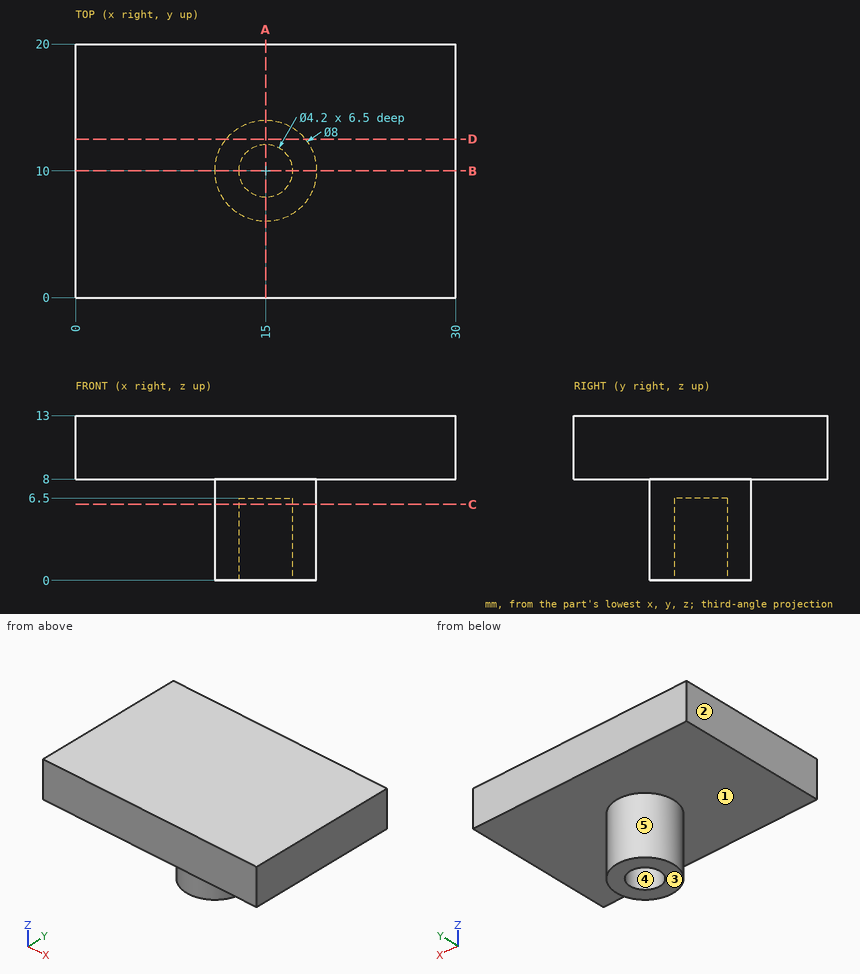
Source: three-view drawing plus pictorial views. Frame: mm from the lowest corner of the part. A direction names the side the tool comes from. Coordinates: 2 decimals unless noted, no trailing zeros. Order: outer loops, then holes, each group sorted by start corner. A loop starts at its lowest first (then second) coordinate and runs counter-clockwise, first axis right, second up.
1) Ray query, probe 1 along Y at (x, z) = (15, 4.5); probe 2 along Z at (x, y) = (22.5, 7.75); probe 3 along Z at (x, y) = (15, 10.5). Return the intervals inside material, ascending.
Result sheet:
probe 1: y = 6 to 7.9, 12.1 to 14
probe 2: z = 8 to 13
probe 3: z = 6.5 to 13
2) Section C-C (z = 6). Return loops of the section in (x, y).
Result sheet:
outline: circle Ø8 at (15, 10); hole circle Ø4.2 at (15, 10)
3) Section B-B (y = 10). Return loops of the section in (x, z), then the cut area to 3 significant figures.
Result sheet:
outline: (0, 8) - (11, 8) - (11, 0) - (12.9, 0) - (12.9, 6.5) - (17.1, 6.5) - (17.1, 0) - (19, 0) - (19, 8) - (30, 8) - (30, 13) - (0, 13) - close
area: 187 mm2
4) Draft query along Y for the marked faces 3, 4 and 5. Return one class per face: released by +Y, released by -Y, zero draft, split by the parting line, or undercut.
Result sheet:
face 3: zero draft
face 4: undercut
face 5: split by the parting line
5) Set-up query: the marked faces 1 and 2. Return all of +Z, -Z, +X, -X, +Y, -Y with unobstructed straight access to the full face (end or side cutting, diameter ignored); none if empty.
Result sheet:
face 1: -Z
face 2: +Z, -Z, -X, +Y, -Y
6) Section A-A (x = 15). Return loops of the section in (y, z), then the cut area to 3 significant figures.
Result sheet:
outline: (0, 8) - (6, 8) - (6, 0) - (7.9, 0) - (7.9, 6.5) - (12.1, 6.5) - (12.1, 0) - (14, 0) - (14, 8) - (20, 8) - (20, 13) - (0, 13) - close
area: 137 mm2
7) First-contact query: P1, Ø5, axis at x = 8, z = 7.5, coming from the -Y side; P2, Ø2, axis at y = 14.5, z = 3.5, coming from the +X side; P3, Ø1, axis at x = 3.5, y = 2, coming from the -Z side; P4, Ø3.5, axis at x = 15, y = 10, coming from the -Z side. Flat tips, straight axial feed; report the tip coordinate or a pass-through.
Result sheet:
P1: stops at y = 0
P2: stops at x = 16.94
P3: stops at z = 8
P4: stops at z = 6.5
8) Section D-D (y = 12.5). Return loops of the section in (x, z), then the cut area to 3 significant figures.
Result sheet:
outline: (0, 8) - (11.88, 8) - (11.88, 0) - (18.12, 0) - (18.12, 8) - (30, 8) - (30, 13) - (0, 13) - close
area: 200 mm2
